Design review of the part built by this model. Coordinates are the model's own, in mm. Coordinates: 2 decimals unless noted, no trailing zeros. Write each loop counter-clockwise with the first axis right and the second up, starting at its lowest first coordinate (ties: lowest second). Pieces come first, ordered by that corner, then holes.
Q1. Add section A-A, the plane x = 30.5. Give the boundary of the cut face in (y, z).
Q2. To check wall thickness, follow probe 1 along X at (y, z) = (23.5, 6.25) (3 decimals); probe 2 along X at (y, z) = (16.35, 3.5) (3 decimals); probe 3 along X at (y, z) = (106, 2.25) (3 decimals). State the ranges of each line that lie inside material, in increasing order.
Q3. Add section C-C, the plane z = 4.25. Give the number of separate pieces and of enclosed holes in the cut face, plus the area to 3 significant figures.
Q4. Add section B-B, the plane y = 61. Give the boundary of the cut face in (x, z) (3 decimals).
Q5. Clearance check with flat-ended pins moving along their axes: pin 1 Ø3 at (x, z) = (-185.5, 2.5) entering from -Y; pin 2 Ø3.5 at (x, y) = (158.375, -19.35) entering from -Z; pin 3 Ø1 at (x, z) = (-93, 2) entering from +Y; pin 4 Ø1.9 at (x, z) = (73.5, 3.5) entering from +Y. State where each tip first meets the part, or that it passes through.
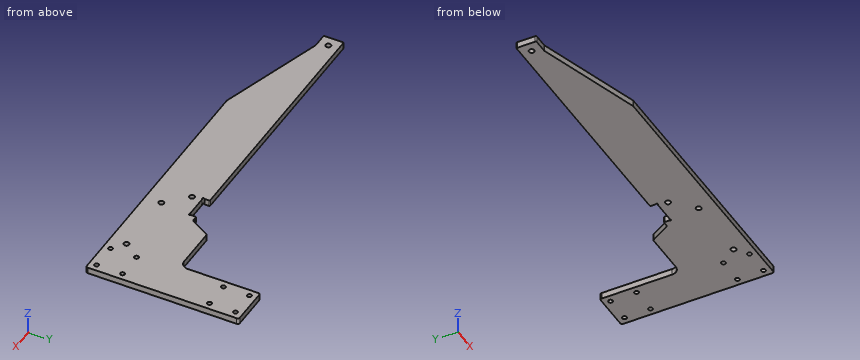
Autodesk Inventor part; units mm, degrees
ref_plane "YZ Plane" through (0, 0, 0) normal (1, 0, 0) x (0, 1, 0)
ref_plane "XZ Plane" through (0, 0, 0) normal (0, 1, 0) x (-1, 0, 0)
ref_plane "XY Plane" through (0, 0, 0) normal (0, 0, 1) x (1, 0, 0)
sketch "Sketch1" plane through (0, 0, 0) normal (0, 0, 1) x (1, 0, 0)
  line L0 (191.375, -26.35) -> (-191.375, -26.35)
  line L1 (-191.375, -26.35) -> (-191.375, 26.35)
  line L2 (-191.375, 26.35) -> (191.375, 26.35)
  line L3 (191.375, 26.35) -> (191.375, -26.35)
  line L4 (191.375, -26.35) -> (-191.375, 26.35) construction
  line L5 (-191.375, -26.35) -> (191.375, 26.35) construction
  line L6 (-191.375, 26.35) -> (-171.375, 26.35)
  line L7 (-171.375, 26.35) -> (-171.375, 6.35)
  line L8 (-171.375, 6.35) -> (-191.375, 6.35)
  line L9 (-191.375, 6.35) -> (-191.375, 26.35)
  line L10 (-176.375, 6.35) -> (-71.375, -26.35)
  line L11 (-181.375, 6.35) -> (-181.375, 46.2875) construction
  line L12 (71.125, 20) -> (91.125, 20)
  line L13 (91.125, 20) -> (91.125, -20)
  line L14 (91.125, -20) -> (71.125, -20)
  line L15 (71.125, -20) -> (71.125, 20)
  line L16 (-190.125, 46.2875) -> (79.875, 46.2875) construction
  line L17 (79.875, 46.2875) -> (79.875, 38.35) construction
  line L18 (79.875, 38.35) -> (-190.125, 38.35) construction
  line L19 (-190.125, 38.35) -> (-190.125, 46.2875) construction
  line L20 (71.125, 46.2875) -> (-181.375, 46.2875) construction
  line L21 (191.375, -26.35) -> (151.375, -26.35)
  line L22 (151.375, -26.35) -> (151.375, 13.65)
  line L23 (151.375, 13.65) -> (191.375, 13.65)
  line L24 (191.375, 13.65) -> (191.375, -26.35)
  line L25 (191.375, -26.35) -> (151.375, 13.65) construction
  line L26 (151.375, -26.35) -> (191.375, 13.65) construction
  line L27 (184.375, -19.35) -> (158.375, -19.35) construction
  line L28 (158.375, -19.35) -> (158.375, 6.65) construction
  line L29 (158.375, 6.65) -> (184.375, 6.65) construction
  line L30 (184.375, 6.65) -> (184.375, -19.35) construction
  line L31 (184.375, -19.35) -> (158.375, 6.65) construction
  line L32 (158.375, -19.35) -> (184.375, 6.65) construction
  line L33 (191.375, 86.65) -> (151.375, 86.65)
  line L34 (151.375, 86.65) -> (151.375, 126.65)
  line L35 (151.375, 126.65) -> (191.375, 126.65)
  line L36 (191.375, 126.65) -> (191.375, 86.65)
  line L37 (191.375, 86.65) -> (151.375, 126.65) construction
  line L38 (151.375, 86.65) -> (191.375, 126.65) construction
  line L39 (184.375, 93.65) -> (158.375, 93.65) construction
  line L40 (158.375, 93.65) -> (158.375, 119.65) construction
  line L41 (158.375, 119.65) -> (184.375, 119.65) construction
  line L42 (184.375, 119.65) -> (184.375, 93.65) construction
  line L43 (184.375, 93.65) -> (158.375, 119.65) construction
  line L44 (158.375, 93.65) -> (184.375, 119.65) construction
  line L45 (191.375, 86.65) -> (191.375, 26.35)
  line L46 (151.375, 86.65) -> (151.375, 13.65)
  line L47 (171.375, -6.35) -> (211.375, -6.35) construction
  line L48 (-181.375, 26.3188) -> (-181.375, 6.35) construction
  line L49 (156.125, -20) -> (136.125, -20)
  line L50 (136.125, -20) -> (136.125, 0)
  line L51 (136.125, 0) -> (156.125, 0)
  line L52 (156.125, 0) -> (156.125, -20)
  line L53 (156.125, -20) -> (136.125, 0) construction
  line L54 (136.125, -20) -> (156.125, 0) construction
  line L55 (91.125, 20) -> (51.125, 20)
  line L56 (51.125, 20) -> (51.125, 0)
  line L57 (51.125, 0) -> (91.125, 0)
  line L58 (91.125, 0) -> (91.125, 20)
  line L59 (151.375, 46.35) -> (101.375, 46.35)
  line L60 (101.375, 46.35) -> (89.828, 26.35)
  point P0 (0, 0)
  point P1 (71.125, 0)
  point P2 (-55.125, 46.2875)
  point P3 (171.375, 106.65)
  point P4 (116.734, 26.35)
  point P5 (61.125, 10)
  point P6 (81.125, -10)
  point P7 (91.125, 0)
  point P8 (88.5805, 0)
  point P9 (81.125, 20)
  point P10 (146.125, -10)
  point P11 (146.125, -10)
  point P12 (51.125, 10)
  point P13 (81.125, -20)
  point P14 (-181.375, 16.35)
  point P15 (-191.375, 16.35)
  point P16 (-171.375, 26.35)
  point P17 (151.375, 26.35)
  dimension "d0" = 52.7
  dimension "d1" = 20
  dimension "d2" = 20
  dimension "d4" = 120
  dimension "d5" = 20
  dimension "d6" = 40
  dimension "d8" = 270
  dimension "d9" = 7.9375
  dimension "d10" = 12
  dimension "d11" = 40
  dimension "d12" = 40
  dimension "d13" = 26
  dimension "d14" = 26
  dimension "d15" = 40
  dimension "d16" = 40
  dimension "d17" = 26
  dimension "d18" = 26
  dimension "d19" = 153
  dimension "d20" = 40
  dimension "d21" = 226.5
  dimension "d22" = 15
  dimension "d35" = 20
  dimension "d47" = 20
  dimension "d48" = 20
  dimension "d49" = 45
  dimension "d57" = 252.5
  dimension "d58" = 10
  dimension "d59" = 10
  dimension "d69" = 120
  dimension "d70" = 50
extrude "Extrusion1" add sketch "Sketch1" along normal blind 6.35 contours L0 L22 L49 L52 L51 L23 L3 | L0 L10 L8 L7 L2 L46 L22 L51 L50 L49 | L23 L46 L2 L3 | L49 L50 L51 L22 | L22 L51 L52 L49 | L2 L46 L33 L45 | L8 L1 L2 L7 | L2 L60 L59 L46 | L33 L34 L35 L36 | L12 L13 L57 L15 | L15 L57 L56 L55 | L57 L13 L14 L15
fillet "Fillet2" radius 1 2 edges at (-191.375, 26.35, 3.175) (-191.375, 6.35, 3.175)
fillet "Fillet5" radius 8 1 edges at (151.375, 46.35, 3.175)
fillet "Fillet3" radius 2 7 edges at (151.375, 126.65, 3.175) (191.375, 126.65, 3.175) (191.375, -26.35, 3.175) (89.828, 26.35, 3.175) (101.375, 46.35, 3.175) (-71.375, -26.35, 3.175) (-176.375, 6.35, 3.175)
hole "Hole1" at (61.125, 10, 0) at (81.125, -10, 0) at (146.125, -10, 0) at (-181.375, 16.35, 0) direction (0, 0, 1) diameter 5.3 end through all
hole "Hole2" at (184.375, 6.65, 0) at (158.375, 6.65, 0) at (158.375, -19.35, 0) at (184.375, -19.35, 0) at (184.375, 119.65, 0) at (158.375, 119.65, 0) at (158.375, 93.65, 0) at (184.375, 93.65, 0) direction (0, 0, 1) diameter 4.3 end through all
sketch "Sketch2" plane through (0, 0, 6.35) normal (0, 0, 1) x (1, 0, 0)
  line L0 (83.875, 19.5) -> (58.375, 19.5)
  line L1 (58.375, 19.5) -> (58.375, 26.35)
  line L2 (58.375, 26.35) -> (83.875, 26.35)
  line L3 (83.875, 26.35) -> (83.875, 19.5)
  line L4 (83.875, 19.5) -> (58.375, 26.35) construction
  line L5 (58.375, 19.5) -> (83.875, 26.35) construction
  circle A0 centre (61.125, 10) radius 2.65
  circle A1 centre (81.125, -10) radius 2.65
  line L6 (61.125, 10) -> (81.125, -10) construction
  line L7 (88.6733, 26.35) -> (-190.375, 26.35) construction
  circle A2 centre (58.775, 19.9) radius 0.9
  circle A3 centre (83.475, 19.9) radius 0.9
  line L8 (83.475, 25.95) -> (58.775, 25.95) construction
  line L9 (58.775, 25.95) -> (58.775, 19.9) construction
  line L10 (58.775, 19.9) -> (83.475, 19.9) construction
  line L11 (83.475, 19.9) -> (83.475, 25.95) construction
  line L12 (83.475, 25.95) -> (58.775, 19.9) construction
  line L13 (58.775, 25.95) -> (83.475, 19.9) construction
  point P0 (0, 0)
  point P1 (71.125, 22.925)
  point P2 (71.125, 0)
  point P3 (119.4481, 26.35)
  point P4 (58.375, 20.7062)
  point P5 (59.5812, 19.5)
  point P6 (82.6688, 19.5)
  point P7 (83.875, 20.7062)
  point P8 (194.625, 26.35)
  point P9 (154.625, 26.35)
  point P10 (93.078, 26.35)
  dimension "d60" = 25.5
  dimension "d61" = 6.85
  dimension "d62" = 1.8
  dimension "d63" = 0.4
  dimension "d64" = 0.4
extrude "Extrusion2" cut sketch "Sketch2" against normal through all contours L3 A3 L0 | L0 A3 L3 | L0 A2 L1 L2 L3 A3 | A2 L1 L0 | L0 L1 A2
fillet "Fillet4" radius 1 6 edges at (83.875, 20.7062, 3.175) (82.6688, 19.5, 3.175) (59.5812, 19.5, 3.175) (58.375, 20.7062, 3.175) (58.375, 26.35, 3.175) (83.875, 26.35, 3.175)
properties part number "Z-Axis Support Plates" material "Aluminum 6061"
Here are the results:
1. outline: (-26.35, 0) - (26.35, 0) - (26.35, 6.35) - (-26.35, 6.35) - close
2. probe 1: x = -191.375 to 58.375, 83.875 to 191.375
2. probe 2: x = -191.375 to -184.025, -178.725 to 191.375
2. probe 3: x = 151.375 to 191.375
3. separate pieces: 1
3. enclosed holes: 12
3. area: 22,700 mm2
4. outline: (151.375, 0) - (191.375, 0) - (191.375, 6.35) - (151.375, 6.35) - close
5. pin 1: stops at y = 6.35
5. pin 2: passes through
5. pin 3: stops at y = 26.35
5. pin 4: stops at y = 19.5
